from build123d import *

# Parameters (mm, degrees)
SKETCH1_R           = 2.4
BOSS_EXTRUDE1_DEPTH = 3.9
SKETCH2_R           = 3.05
CUT_EXTRUDE1_DEPTH  = 0.8
SKETCH3_R           = 3.05
CUT_EXTRUDE2_DEPTH  = 0.8


with BuildPart() as part:
    # Sketch1 → Boss-Extrude1 (new body)
    with BuildSketch(Plane(origin=(0, 0, 0), x_dir=(1, 0, 0), z_dir=(0, 1, 0))):
        with BuildLine():
            Line((-12.035, 3.65), (12.035, 3.65))
            ThreePointArc((12.035, 3.65), (15.685, 0), (12.035, -3.65))
            Line((12.035, -3.65), (-12.035, -3.65))
            ThreePointArc((-12.035, -3.65), (-15.685, 0), (-12.035, 3.65))
        make_face()
        with Locations((-4.033060202, 0.018008222)):
            Circle(SKETCH1_R, mode=Mode.SUBTRACT)
        with Locations((4.035, 0.008270612)):
            Circle(SKETCH1_R, mode=Mode.SUBTRACT)
        Polygon((11.135, 2.4), (11.135, 0.9), (9.635, 0.9), (9.635, -0.9), (11.135, -0.9), (11.135, -2.4), (12.935, -2.4), (12.935, -0.9), (14.435, -0.9), (14.435, 0.9), (12.935, 0.9), (12.935, 2.4), align=None, mode=Mode.SUBTRACT)
        Polygon((-12.933060202, 2.401087844), (-12.933060202, 0.901087844), (-14.433060202, 0.901087844), (-14.433060202, -0.898912156), (-12.933060202, -0.898912156), (-12.933060202, -2.398912156), (-11.133060202, -2.398912156), (-11.133060202, -0.898912156), (-9.633060202, -0.898912156), (-9.633060202, 0.901087844), (-11.133060202, 0.901087844), (-11.133060202, 2.401087844), align=None, mode=Mode.SUBTRACT)
    extrude(amount=BOSS_EXTRUDE1_DEPTH)

    # Sketch2 → Cut-Extrude1 (cut)
    with BuildSketch(Plane(origin=(0, 3.9, 0), x_dir=(1, 0, 0), z_dir=(0, 1, 0))):
        with Locations((4.035, 0.008270612)):
            Circle(SKETCH2_R)
        with Locations((-4.033060202, 0.018008222)):
            Circle(SKETCH2_R)
    extrude(amount=-CUT_EXTRUDE1_DEPTH, mode=Mode.SUBTRACT)

    # Sketch3 → Cut-Extrude2 (cut)
    with BuildSketch(Plane(origin=(0, 0, 0), x_dir=(-1, 0, 0), z_dir=(0, -1, 0))):
        with Locations((4.033060202, 0.018008222)):
            Circle(SKETCH3_R)
        with Locations((-4.035, 0.008270612)):
            Circle(SKETCH3_R)
    extrude(amount=-CUT_EXTRUDE2_DEPTH, mode=Mode.SUBTRACT)


solid = part.part
The model under review builds one solid part; all positions refer to its coordinate system, in mm. A direction names the side the tool comes from. Give positions to 0.01 mm unless a question says otherwise; leave off trailing zeros. Loops run counter-clockwise (first coordinate to the right, second up) from the corner with the lowest first, then second, coordinate; pieces in that order, holes last. Notation, with made-up numbers: (-11.75, 11.25) -> (6.25, 11.25) arc R15 cw to (6.25, 27.25) -> close; hole circle Ø6 at (28, 47.5). An arc over 180 degrees is marked (long way). Write each question's results on one line, items separated by ' | '.
1) Tool access review of faces 4 (the face through (-15.684, 1.923, 0.08)), 5 (the face through (6, 0.8, 2)), 6 (the face through (0.988, 3.506, -0.142)), 7 (the face through (-11.133, 2, -2)): name each direction out of +Z, -Z, +X, -X, +Y, -Y from which nothing blocks a thin tool from reaching the whole face with its end or side.
Conclusion:
face 4: -X, +Y, -Y | face 5: -Y | face 6: +Y | face 7: +Y, -Y
2) For line 1 along X through (y, z) = (0.25, -1.25) (3 decimals); line 2 along X through (y, z) = (2, -1.75) (3 decimals); line 3 along Y through (x, z) = (7, 0), list the stretches that pass through material, from the lowest coordinate up. Write a range as from..to.
Conclusion:
line 1: x = -15.464..-12.933, -11.133..-6.823, -1.243..1.249, 6.821..11.135, 12.935..15.464 | line 2: x = -15.238..-12.933, -11.133..-5.694, -2.372..2.384, 5.686..11.135, 12.935..15.238 | line 3: y = 0.8..3.1
3) Take a section at A-A, the plane y = 1.5. Count the separate pieces of the cut face and the enclosed holes in it, plus the area to 3 significant figures.
Conclusion:
separate pieces: 1 | enclosed holes: 4 | area: 153 mm^2
4) Take a section at B-B, the plane x = 5.5. Give the boundary of the cut face in (y, z).
Conclusion:
outline: (0, -3.65) -> (3.9, -3.65) -> (3.9, -2.68) -> (3.1, -2.68) -> (3.1, -1.91) -> (0.8, -1.91) -> (0.8, -2.68) -> (0, -2.68) -> close; (0, 2.67) -> (0.8, 2.67) -> (0.8, 1.89) -> (3.1, 1.89) -> (3.1, 2.67) -> (3.9, 2.67) -> (3.9, 3.65) -> (0, 3.65) -> close
5) Insertion check: pin 1 Ø0.8 at (y, z) = (1, 1.5) entering from -X; pin 2 Ø0.8 at (y, z) = (2, -1.5) entering from +X; pin 3 Ø1.2 at (y, z) = (2, 2) entering from +X; pin 4 Ø1.8 at (x, z) = (-3.5, 1) entering from +Y. Each pin has a flat end and moves straight along its axis. Give the tip position at first contact, or say it passes through.
Conclusion:
pin 1: stops at x = -15.52 | pin 2: stops at x = 15.52 | pin 3: stops at x = 15.41 | pin 4: passes through
6) Draft analysis for pull direction Z (two halves, no side actions). For faces 1 (the face through (0, 2, -3.65)), 2 (the face through (0, 3.9, 0)), 3 (the face through (-10, 2, -0.901)), state which applies: pulls with the +Z half, pulls with the -Z half, needs draft (parallel to the pull), parting line crosses it, or undercut.
Conclusion:
face 1: pulls with the -Z half | face 2: needs draft | face 3: undercut
